```python
from build123d import *

# Parameters (mm, degrees)
BASE_FLANGE1_DEPTH      = 60.325
CUT_EXTRUDE1_DEPTH      = 83.467433131
CUT_EXTRUDE1_DEPTH_BACK = 83.467433131
SKETCH6_R               = 2.4892


# Sheet-metal steps are written as plain solids
with BuildPart() as part:
    # Sketch1 → Base-Flange1 (new body)
    with BuildSketch(Plane.XY):
        with BuildLine():
            Line((-53.2765, -6.35), (-53.2765, 5.588))
            ThreePointArc((-53.2765, 5.588), (-53.053315367, 6.126815367), (-52.5145, 6.35))
            Line((-52.5145, 6.35), (52.5145, 6.35))
            ThreePointArc((52.5145, 6.35), (53.053315367, 6.126815367), (53.2765, 5.588))
            Line((53.2765, 5.588), (53.2765, -6.35))
            Line((53.2765, -6.35), (55.5625, -6.35))
            Line((55.5625, -6.35), (55.5625, 5.588))
            ThreePointArc((55.5625, 5.588), (54.669761469, 7.743261469), (52.5145, 8.636))
            Line((52.5145, 8.636), (-52.5145, 8.636))
            ThreePointArc((-52.5145, 8.636), (-54.669761469, 7.743261469), (-55.5625, 5.588))
            Line((-55.5625, 5.588), (-55.5625, -6.35))
            Line((-55.5625, -6.35), (-53.2765, -6.35))
        make_face()
    extrude(amount=BASE_FLANGE1_DEPTH)

    # Sketch6 → Cut-Extrude1 (cut, two sides: drawn at the far end of the back side and taken through both)
    with BuildSketch(Plane(origin=(0, 0, 0), x_dir=(0, 0, -1), z_dir=(1, 0, 0)).offset(-CUT_EXTRUDE1_DEPTH_BACK)):
        with Locations((-30.1625, -0.92202)):
            Circle(SKETCH6_R)
        with Locations((-20.32, -0.92202)):
            Circle(SKETCH6_R)
        with Locations((-7.62, -0.92202)):
            Circle(SKETCH6_R)
        with Locations(Location((-52.705, -0.92202, 0), (0, 0, 180))):
            Circle(SKETCH6_R)
        with Locations(Location((-40.005, -0.92202, 0), (0, 0, 180))):
            Circle(SKETCH6_R)
    extrude(amount=CUT_EXTRUDE1_DEPTH + CUT_EXTRUDE1_DEPTH_BACK, mode=Mode.SUBTRACT)


solid = part.part
```
Input: part model. Units: mm. Frame: model coordinates. A direction names the side the tool comes from. Give positions to 0.01 mm unless a question says otherwise; leave off trailing zeros. Order: outer loops, then holes, each group sorted by start corner. A loop starts at its lowest first (then second) coordinate and runs counter-clockwise, first axis right, second up. Notation, with made-up numbers: (23, 39.5) - (29, 39.5) arc R28 ccw to (29, 70.5) - close; hole circle Ø11 at (73.5, 28.25). An arc over 180 degrees is marked (long way). Use a Markdown table: item, result.
(1) Section query C-C (z = 49). Output: boundary loops of the cut face in (x, y).
Computed values:
| item | result |
|---|---|
| outline | (-55.56, -6.35) - (-53.28, -6.35) - (-53.28, 5.59) arc R0.76 cw to (-52.51, 6.35) - (52.51, 6.35) arc R0.76 cw to (53.28, 5.59) - (53.28, -6.35) - (55.56, -6.35) - (55.56, 5.59) arc R3.05 ccw to (52.51, 8.64) - (-52.51, 8.64) arc R3.05 ccw to (-55.56, 5.59) - close |
(2) Line query: line 1 (X direction, y = 3, z = 22); line 2 (Y direction, x = -41, z = 22); line 3 (Y direction, x = 54, z = 7). Output: solid intervals per line, ascending. Write a range as from..to.
Computed values:
| item | result |
|---|---|
| line 1 | x = -55.56..-53.28, 53.28..55.56 |
| line 2 | y = 6.35..8.64 |
| line 3 | y = -6.35..-3.33, 1.49..8.25 |
(3) Access query for faces 4 (the cylindrical face through (-54.436, -0.174, 17.946)), 5 (the flat face through (53.276, 2, 30)). Directions: +Z, -Z, +X, -X, +Y, -Y. A direction counts if a zero-diameter tool reaches every point of the face in a straight line with its end or side. Return the directions, or none.
Computed values:
| item | result |
|---|---|
| face 4 | +X, -X |
| face 5 | +Z, -Z, -Y |
(4) Section query B-B (y = 3). Output: boundary loops of the cut face in (x, z) (1 decimal), then the cut area to 3 significant figures.
Computed values:
| item | result |
|---|---|
| outline | (-55.6, 0) - (-53.3, 0) - (-53.3, 60.3) - (-55.6, 60.3) - close; (53.3, 0) - (55.6, 0) - (55.6, 60.3) - (53.3, 60.3) - close |
| area | 276 mm2 |
(5) Draft query along Y for faces 1 (the flat face through (-53.276, 2, 30)), 2 (the flat face through (-1, 6.35, 30)), 3 (the cylindrical face through (54.403, -1.875, 5.321)). Return one class per face: released by +Y, released by -Y, zero draft, split by the parting line, or undercut.
Computed values:
| item | result |
|---|---|
| face 1 | zero draft |
| face 2 | released by -Y |
| face 3 | undercut |
(6) Section query D-D (x = -40). Output: boundary loops of the cut face in (y, z) (3 decimals), then the cut area to 3 significant figures.
Computed values:
| item | result |
|---|---|
| outline | (6.35, 0) - (8.636, 0) - (8.636, 60.325) - (6.35, 60.325) - close |
| area | 138 mm2 |
(7) Section query A-A (z = 7.62). Output: boundary loops of the cut face in (x, y).
Computed values:
| item | result |
|---|---|
| outline | (-55.56, -6.35) - (-53.28, -6.35) - (-53.28, -3.41) - (-55.56, -3.41) - close; (-55.56, 1.57) - (-53.28, 1.57) - (-53.28, 5.59) arc R0.76 cw to (-52.51, 6.35) - (52.51, 6.35) arc R0.76 cw to (53.28, 5.59) - (53.28, 1.57) - (55.56, 1.57) - (55.56, 5.59) arc R3.05 ccw to (52.51, 8.64) - (-52.51, 8.64) arc R3.05 ccw to (-55.56, 5.59) - close; (53.28, -6.35) - (55.56, -6.35) - (55.56, -3.41) - (53.28, -3.41) - close |
(8) Pin query (flat end, axial travel): pin 1 (4 mm diameter, centred on y = -0.92, z = 52.7, fed in from +X); pin 2 (6 mm diameter, centred on x = -12, z = 52, fed in from -Y). Return the tip coordinate at first contact, or that it passes through.
Computed values:
| item | result |
|---|---|
| pin 1 | passes through |
| pin 2 | stops at y = 6.35 |
